Could you check a few things on this model? Use its own coordinates, in mm. A direction names the side the tool comes from. Coordinates: 2 decimals unless noted, no trailing zeros. Loops run counter-clockwise (first coordinate to the right, second up) from the corner with the lowest first, then second, coordinate; pieces in that order, holes last. Notation, with made-up numbers: (-38.5, -14) - (-2.5, -14) arc R24 cw to (-2.5, 15) - close; hole circle Ø11 at (-22, 81). An arc over 180 degrees is marked (long way). Use CSV: the item, a comma, the result in double quotes.
from build123d import *

# Parameters (mm, degrees)
F0_W     = 228.6
F0_H     = 292.1
F1_DEPTH = 38.1
F2_W     = 215.9
F2_H     = 25.4
F3_DEPTH = 279.4
F4_R     = 31.202064
F5_DEPTH = 6.35
F6_R     = 7.745315
F7_DEPTH = 6.35


with BuildPart() as f1:
    # F0 (on Top) → F1 (new body)
    with BuildSketch(Plane.XY):
        with Locations((0.30422, -19.358111)):
            Rectangle(F0_W, F0_H)
    extrude(amount=F1_DEPTH)

    # F2 (on face) → F3 (cut)
    with BuildSketch(Plane(origin=(0, 126.691889, 0), x_dir=(-1, 0, 0), z_dir=(0, 1, 0))):
        with Locations((-0.30422, 19.05)):
            Rectangle(F2_W, F2_H)
    extrude(amount=-F3_DEPTH, mode=Mode.SUBTRACT)

    # F4 (on face) → F5 (cut)
    with BuildSketch(Plane.XY.offset(38.1)):
        with Locations((0.30422, 126.691889)):
            Circle(F4_R)
    extrude(amount=-F5_DEPTH, mode=Mode.SUBTRACT)

    # F6 (on face) → F7 (cut)
    with BuildSketch(Plane(origin=(0, 0, 0), x_dir=(1, 0, 0), z_dir=(0, 0, -1))):
        with Locations((-63.446887, 114.401668)):
            Circle(F6_R)
        with Locations((-63.446887, 12.801668)):
            Circle(F6_R)
        with Locations((-63.446887, -88.798332)):
            Circle(F6_R)
        with Locations((63.553113, 114.401668)):
            Circle(F6_R)
        with Locations((63.553113, 12.801668)):
            Circle(F6_R)
        with Locations((63.553113, -88.798332)):
            Circle(F6_R)
    extrude(amount=-F7_DEPTH, mode=Mode.SUBTRACT)


solid = f1.part
(1) Suppose I cut it at A-A (y = 54.5). Write out the boundary of the cut face in (x, z), plus the area to 3 significant figures.
Computed:
outline,"(-114, 0) - (114.6, 0) - (114.6, 38.1) - (-114, 38.1) - close; hole (-107.65, 6.35) - (108.25, 6.35) - (108.25, 31.75) - (-107.65, 31.75) - close"
area,"3,230 mm²"
(2) Thinking about a two-plate mould opening in Z: for faces 1 (the face through (-1, -17, 0)), 2 (the face through (-1, -17, 38.1)), 3 (the face through (-1, -165.408, 19)), 4 (the face through (2, -11, 6.35)), which applies, +Z half, -Z half, draft (parallel to the pull), parting line (faces both ways), or undercut?
Computed:
face 1,"-Z half"
face 2,"+Z half"
face 3,"draft"
face 4,"undercut"
(3) Please list where these lines run through material, in increasing order: line 1 (X direction, y = 88.5, z = 4); line 2 (Z direction, x = -25, y = 60); line 3 (X direction, y = -87, z = 27.5).
Computed:
line 1,"x = -114 to -71.19, -55.71 to 55.81, 71.29 to 114.6"
line 2,"z = 0 to 6.35, 31.75 to 38.1"
line 3,"x = -114 to -107.65, 108.25 to 114.6"
(4) Will these pins go through, and if not, where does the flat tip stop? pin 1 (14 mm diameter, centred on x = 63.55, y = -12.8, fed in from -Z); pin 2 (20.5 mm diameter, centred on x = 42, z = 17, fed in from +Y).
Computed:
pin 1,"stops at z = 31.75"
pin 2,"stops at y = -152.71"
(5) Suppose I cut it at D-D (z = 3). Write out the boundary of the cut face in (x, y).
Computed:
outline,"(-114, -165.41) - (114.6, -165.41) - (114.6, 126.69) - (-114, 126.69) - close; hole circle Ø15.49 at (-63.45, -114.4); hole circle Ø15.49 at (-63.45, -12.8); hole circle Ø15.49 at (-63.45, 88.8); hole circle Ø15.49 at (63.55, -114.4); hole circle Ø15.49 at (63.55, -12.8); hole circle Ø15.49 at (63.55, 88.8)"
(6) Suppose I cut it at C-C (z = 28.5). Write out the boundary of the cut face in (x, y).
Computed:
outline,"(-114, -165.41) - (114.6, -165.41) - (114.6, 126.69) - (108.25, 126.69) - (108.25, -152.71) - (-107.65, -152.71) - (-107.65, 126.69) - (-114, 126.69) - close"
(7) Suppose I cut it at B-B (x = 99). Write out the boundary of the cut face in (y, z), plus the area to 3 significant figures.
Computed:
outline,"(-165.41, 0) - (126.69, 0) - (126.69, 6.35) - (-152.71, 6.35) - (-152.71, 31.75) - (126.69, 31.75) - (126.69, 38.1) - (-165.41, 38.1) - close"
area,"4,030 mm²"
(8) Which directions (+Z, -Z, +X, -X, +Y, -Y) give clear straight access to the entire face, cutting with the end or side of a thin tool? Please do faces 5 (the face through (0, 126.692, 6)), 6 (the face through (-107.646, -11, 19)), 7 (the face through (-0.382, 95.497, 34.969)), 8 (the face through (-59.87, 95.67, 3.13)).
Computed:
face 5,"+Z, -Z, +X, -X, +Y"
face 6,"+Y"
face 7,"+Z, +Y"
face 8,"-Z"
